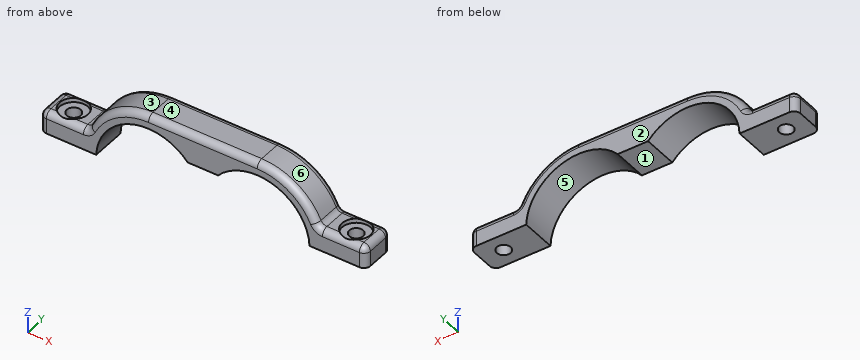
from build123d import *

# Parameters (mm, degrees)
BOSS_EXTRU_1_DEPTH      = 8
ESQUISSE2_R             = 1.6
ENL_V_MAT_EXTRU_1_DEPTH = 42.011614209
ENL_V_START             = -4
ESQUISSE3_R             = 3.25
ENL_V_MAT_EXTRU_2_DEPTH = 38.011614209
CONG_1_R                = 1.5


with BuildPart() as part:
    # Esquisse1 → Boss.-Extru.1 (new body)
    with BuildSketch(Plane(origin=(0, 0, 0), x_dir=(1, 0, 0), z_dir=(0, 1, 0))):
        with BuildLine():
            Line((-37.5, -0.5), (-24.539622087, -0.5))
            ThreePointArc((-24.539622087, -0.5), (-16.544164933, -11.351089375), (-3.488757022, -8))
            Line((-3.488757022, -8), (3.488757022, -8))
            ThreePointArc((3.488757022, -8), (16.544164933, -11.351089375), (24.539622087, -0.5))
            Line((24.539622087, -0.5), (37.5, -0.5))
            Line((37.5, -0.5), (37.5, -5.5))
            Line((37.5, -5.5), (26.509014955, -5.5))
            ThreePointArc((26.509014955, -5.5), (20.977248964, -12.435382986), (12.5, -15.05))
            Line((12.5, -15.05), (-12.5, -15.05))
            ThreePointArc((-12.5, -15.05), (-20.977248964, -12.435382986), (-26.509014955, -5.5))
            Line((-26.509014955, -5.5), (-37.5, -5.5))
            Line((-37.5, -5.5), (-37.5, -0.5))
        make_face()
    extrude(amount=BOSS_EXTRU_1_DEPTH)

    # Esquisse2 → Enlèv. mat.-Extru.1 (cut, through all)
    with BuildSketch(Plane(origin=(0, 0, 0.5), x_dir=(-1, 0, 0), z_dir=(0, 0, -1))):
        with Locations((32.5, 4)):
            Circle(ESQUISSE2_R)
        with Locations((-32.5, 4)):
            Circle(ESQUISSE2_R)
    extrude(amount=-ENL_V_MAT_EXTRU_1_DEPTH, mode=Mode.SUBTRACT)

    # Esquisse3 → Enlèv. mat.-Extru.2 (cut, through all)
    with BuildSketch(Plane(origin=(0, 0, 0.5), x_dir=(-1, 0, 0), z_dir=(0, 0, -1)).offset(ENL_V_START)):
        with Locations((32.5, 4)):
            Circle(ESQUISSE3_R)
        with Locations((-32.5, 4)):
            Circle(ESQUISSE3_R)
    extrude(amount=-ENL_V_MAT_EXTRU_2_DEPTH, mode=Mode.SUBTRACT)

    # Congé1
    # the kernel refuses this fillet: 1.5 mm, written as the material it adds along each edge
    with BuildSketch(Plane(origin=(26.509014955, 0, 5.5), x_dir=(-0.3943977660181821, 0, 0.9189398251027471), z_dir=(0, 1, 0))) as cong_1_piece_1:
        with BuildLine():
            CenterArc((0.988849381, 1.499265395), CONG_1_R, 203.228419566, 64.978347937)
            Line((-0.389560356, 0.907668746), (0, 0))
            ThreePointArc((0, 0), (0.470955164, 0.007370535), (0.941910328, 0))
        make_face()
    extrude(amount=8)
    with BuildSketch(Plane(origin=(-26.509014955, 0, 5.5), x_dir=(0.3943977660181821, 0, 0.9189398251027471), z_dir=(0, 1, 0))) as cong_1_piece_2:
        with BuildLine():
            CenterArc((0.988849381, -1.499265395), CONG_1_R, 91.793232497, 64.978347937)
            Line((-0.389560356, -0.907668746), (0, 0))
            ThreePointArc((0, 0), (0.470955164, -0.007370535), (0.941910328, 0))
        make_face()
    extrude(amount=8)
    # the kernel refuses this fillet: 1.5 mm, written as the material it takes off along each edge
    with BuildSketch(Plane(origin=(37.5, 0, -3.25), x_dir=(-1, 0, 0), z_dir=(0, 0, 1)), Plane(origin=(-37.5, 0, 9.25), x_dir=(1, 0, 0), z_dir=(0, 0, -1))) as cong_1_2_piece_1:
        with BuildLine():
            CenterArc((CONG_1_R, -CONG_1_R), CONG_1_R, 90, 90)
            Line((0, -CONG_1_R), (0, 0))
            Line((0, 0), (CONG_1_R, 0))
        make_face()
    extrude(amount=12.5, mode=Mode.SUBTRACT)
    with BuildSketch(Plane(origin=(-37.5, 8, 9.25), x_dir=(1, 0, 0), z_dir=(0, 0, -1)), Plane(origin=(37.5, 8, -3.25), x_dir=(-1, 0, 0), z_dir=(0, 0, 1))) as cong_1_2_piece_2:
        with BuildLine():
            CenterArc((CONG_1_R, CONG_1_R), CONG_1_R, 180, 90)
            Line((0, CONG_1_R), (0, 0))
            Line((0, 0), (CONG_1_R, 0))
        make_face()
    extrude(amount=12.5, mode=Mode.SUBTRACT)
    with BuildSketch(Plane(origin=(37.5, -3.75, 5.5), x_dir=(0, 0, -1), z_dir=(0, 1, 0)), Plane(origin=(-37.5, -3.75, 5.5), x_dir=(1, 0, 0), z_dir=(0, 1, 0))) as cong_1_2_piece_3:
        with BuildLine():
            CenterArc((CONG_1_R, CONG_1_R), CONG_1_R, 180, 90)
            Line((0, CONG_1_R), (0, 0))
            Line((0, 0), (CONG_1_R, 0))
        make_face()
    extrude(amount=15.5, mode=Mode.SUBTRACT)
    # the kernel refuses this fillet: 1.5 mm, written as the material it takes off along each edge
    with BuildSketch(Plane(origin=(36, 6.5, 4), x_dir=(0, 0, 1), z_dir=(0, 1, 0))) as cong_1_3_piece_1_section:
        Polygon((0, 0), (CONG_1_R, 0), (CONG_1_R, CONG_1_R), (0, CONG_1_R), align=None)
    cong_1_3_piece_1 = extrude(amount=CONG_1_R, mode=Mode.PRIVATE)
    cong_1_3_piece_1 = cong_1_3_piece_1 - Plane(origin=(36, 6.5, 4), x_dir=(-0.7071067811865475, 0, -0.7071067811865475), z_dir=(0, 1, 0)) * Sphere(CONG_1_R, mode=Mode.PRIVATE)
    add(cong_1_3_piece_1, mode=Mode.SUBTRACT)
    with BuildSketch(Plane(origin=(-36, 6.5, 4), x_dir=(0, 0, 1), z_dir=(0, 1, 0))) as cong_1_3_piece_2_section:
        Polygon((0, 0), (CONG_1_R, 0), (CONG_1_R, -CONG_1_R), (0, -CONG_1_R), align=None)
    cong_1_3_piece_2 = extrude(amount=CONG_1_R, mode=Mode.PRIVATE)
    cong_1_3_piece_2 = cong_1_3_piece_2 - Plane(origin=(-36, 6.5, 4), x_dir=(0.7071067811865475, 0, -0.7071067811865475), z_dir=(0, 1, 0)) * Sphere(CONG_1_R, mode=Mode.PRIVATE)
    add(cong_1_3_piece_2, mode=Mode.SUBTRACT)
    with BuildSketch(Plane(origin=(-36, 1.5, 4), x_dir=(0, 0, 1), z_dir=(0, -1, 0))) as cong_1_3_piece_3_section:
        Polygon((0, 0), (CONG_1_R, 0), (CONG_1_R, CONG_1_R), (0, CONG_1_R), align=None)
    cong_1_3_piece_3 = extrude(amount=CONG_1_R, mode=Mode.PRIVATE)
    cong_1_3_piece_3 = cong_1_3_piece_3 - Plane(origin=(-36, 1.5, 4), x_dir=(0.7071067811865475, 0, -0.7071067811865475), z_dir=(0, -1, 0)) * Sphere(CONG_1_R, mode=Mode.PRIVATE)
    add(cong_1_3_piece_3, mode=Mode.SUBTRACT)
    with BuildSketch(Plane(origin=(36, 1.5, 4), x_dir=(0, 0, 1), z_dir=(0, -1, 0))) as cong_1_3_piece_4_section:
        Polygon((0, 0), (CONG_1_R, 0), (CONG_1_R, -CONG_1_R), (0, -CONG_1_R), align=None)
    cong_1_3_piece_4 = extrude(amount=CONG_1_R, mode=Mode.PRIVATE)
    cong_1_3_piece_4 = cong_1_3_piece_4 - Plane(origin=(36, 1.5, 4), x_dir=(-0.7071067811865475, 0, -0.7071067811865475), z_dir=(0, -1, 0)) * Sphere(CONG_1_R, mode=Mode.PRIVATE)
    add(cong_1_3_piece_4, mode=Mode.SUBTRACT)
    with BuildSketch(Plane(origin=(36, 0, 5.5), x_dir=(0, 0, -1), z_dir=(-1, 0, 0)), Plane(origin=(-27.496749648, 0, 5.5), x_dir=(0, 0, -1), z_dir=(-1, 0, 0))) as cong_1_3_piece_5:
        with BuildLine():
            CenterArc((CONG_1_R, -CONG_1_R), CONG_1_R, 90, 90)
            Line((0, -CONG_1_R), (0, 0))
            Line((0, 0), (CONG_1_R, 0))
        make_face()
    extrude(amount=8.503250352, mode=Mode.SUBTRACT)
    with BuildSketch(Plane(origin=(12.5, 0, 0), x_dir=(0.9061480149752484, 0, 0.4229607250755286), z_dir=(0.4229607250755286, 0, -0.9061480149752484))) as cong_1_3_piece_6:
        with BuildLine():
            CenterArc((15.05 - CONG_1_R, -CONG_1_R), CONG_1_R, 0, 90)
            Line((15.05 - CONG_1_R, 0), (15.05, 0))
            Line((15.05, 0), (15.05, -CONG_1_R))
        make_face()
    revolve(axis=Axis((12.5, 0, 0), (0, -1, 0)), revolution_arc=64.978347937, mode=Mode.SUBTRACT)
    with BuildSketch(Plane(origin=(12.5, 0, 15.05), x_dir=(0, 0, -1), z_dir=(-1, 0, 0)), Plane(origin=(12.5, 8, 15.05), x_dir=(0, -1, 0), z_dir=(-1, 0, 0))) as cong_1_3_piece_7:
        with BuildLine():
            CenterArc((CONG_1_R, -CONG_1_R), CONG_1_R, 90, 90)
            Line((0, -CONG_1_R), (0, 0))
            Line((0, 0), (CONG_1_R, 0))
        make_face()
    extrude(amount=25, mode=Mode.SUBTRACT)
    with BuildSketch(Plane(origin=(-12.5, 0, 0), x_dir=(0, 0, 1), z_dir=(1, 0, 0))) as cong_1_3_piece_8:
        with BuildLine():
            CenterArc((15.05 - CONG_1_R, -CONG_1_R), CONG_1_R, 0, 90)
            Line((15.05, -CONG_1_R), (15.05, 0))
            Line((15.05, 0), (15.05 - CONG_1_R, 0))
        make_face()
    revolve(axis=Axis((-12.5, 0, 0), (0, -1, 0)), revolution_arc=64.978347937, mode=Mode.SUBTRACT)
    with BuildSketch(Plane(origin=(-27.496749648, 8, 5.5), x_dir=(0, 0, -1), z_dir=(-1, 0, 0)), Plane(origin=(36, 8, 5.5), x_dir=(0, 0, -1), z_dir=(-1, 0, 0))) as cong_1_3_piece_9:
        with BuildLine():
            CenterArc((CONG_1_R, CONG_1_R), CONG_1_R, 180, 90)
            Line((0, CONG_1_R), (0, 0))
            Line((0, 0), (CONG_1_R, 0))
        make_face()
    extrude(amount=8.503250352, mode=Mode.SUBTRACT)
    with BuildSketch(Plane(origin=(-12.5, 8, 0), x_dir=(0, 0, 1), z_dir=(1, 0, 0))) as cong_1_3_piece_10:
        with BuildLine():
            CenterArc((15.05 - CONG_1_R, CONG_1_R), CONG_1_R, 270, 90)
            Line((15.05, CONG_1_R), (15.05, 0))
            Line((15.05, 0), (15.05 - CONG_1_R, 0))
        make_face()
    revolve(axis=Axis((-12.5, 8, 0), (0, -1, 0)), revolution_arc=64.978347937, mode=Mode.SUBTRACT)
    with BuildSketch(Plane(origin=(12.5, 8, 0), x_dir=(0.9061480149752484, 0, 0.4229607250755286), z_dir=(0.4229607250755286, 0, -0.9061480149752484))) as cong_1_3_piece_11:
        with BuildLine():
            CenterArc((15.05 - CONG_1_R, CONG_1_R), CONG_1_R, 270, 90)
            Line((15.05 - CONG_1_R, 0), (15.05, 0))
            Line((15.05, 0), (15.05, CONG_1_R))
        make_face()
    revolve(axis=Axis((12.5, 8, 0), (0, -1, 0)), revolution_arc=64.978347937, mode=Mode.SUBTRACT)
    with BuildSketch(Plane(origin=(27.496749648, 8, 7), x_dir=(-0.9061480149752484, 0, -0.4229607250755287), z_dir=(-0.4229607250755287, 0, 0.9061480149752484))) as cong_1_3_piece_12:
        with BuildLine():
            CenterArc((1.5 + CONG_1_R, CONG_1_R), CONG_1_R, 180, 90)
            Line((1.5, CONG_1_R), (1.5, 0))
            Line((1.5, 0), (1.5 + CONG_1_R, 0))
        make_face()
    revolve(axis=Axis((27.496749648, 8, 7), (0, -1, 0)), revolution_arc=64.978347937, mode=Mode.SUBTRACT)
    with BuildSketch(Plane(origin=(-27.496749648, 8, 7), x_dir=(0.9061480149752487, 0, -0.42296072507552823), z_dir=(0.42296072507552823, 0, 0.9061480149752487))) as cong_1_3_piece_13:
        with BuildLine():
            CenterArc((1.5 + CONG_1_R, -CONG_1_R), CONG_1_R, 90, 90)
            Line((1.5, -CONG_1_R), (1.5, 0))
            Line((1.5, 0), (1.5 + CONG_1_R, 0))
        make_face()
    revolve(axis=Axis((-27.496749648, 8, 7), (0, 1, 0)), revolution_arc=64.978347937, mode=Mode.SUBTRACT)
    with BuildSketch(Plane(origin=(-27.496749648, 0, 7), x_dir=(0.9061480149752487, 0, -0.42296072507552823), z_dir=(0.42296072507552823, 0, 0.9061480149752487))) as cong_1_3_piece_14:
        with BuildLine():
            CenterArc((1.5 + CONG_1_R, CONG_1_R), CONG_1_R, 180, 90)
            Line((1.5, CONG_1_R), (1.5, 0))
            Line((1.5, 0), (1.5 + CONG_1_R, 0))
        make_face()
    revolve(axis=Axis((-27.496749648, 0, 7), (0, 1, 0)), revolution_arc=64.978347937, mode=Mode.SUBTRACT)
    with BuildSketch(Plane(origin=(27.496749648, 0, 7), x_dir=(-0.9061480149752484, 0, -0.4229607250755287), z_dir=(-0.4229607250755287, 0, 0.9061480149752484))) as cong_1_3_piece_15:
        with BuildLine():
            CenterArc((1.5 + CONG_1_R, -CONG_1_R), CONG_1_R, 90, 90)
            Line((1.5, -CONG_1_R), (1.5, 0))
            Line((1.5, 0), (1.5 + CONG_1_R, 0))
        make_face()
    revolve(axis=Axis((27.496749648, 0, 7), (0, -1, 0)), revolution_arc=64.978347937, mode=Mode.SUBTRACT)


solid = part.part
Design review of the part built by this model. Coordinates are the model's own, in mm. Face numbers are marked on the shaded views. A direction names the side the tool comes from. Round coordinates to 2 decimals unless told otherwise and drop trailing zeros. Loops run counter-clockwise (first coordinate to the right, second up) from the corner with the lowest first, then second, coordinate; pieces in that order, holes last. Notation, with made-up numbers: (64.5, 16.25) -> (82.5, 16.25) arc R7 cw to (82.5, 24.25) -> close; hole circle Ø8 at (-35, 51.25). An arc over 180 degrees is marked (long way). Use one line per item in the form item = value. Start each with the question number.
Q1. Machinability: for the marked faces 1 and 2, which of the approach directions +Z, -Z, +X, -X, +Y, -Y give a long, thin tool a straight path to every point of the face, cutting with its end or side? Answer none if there is none.
Q2. Wall thickness on line 1 along X through (y, z) = (1.5, 9.25); line 2 along X through (y, z) = (4, 5.1); line 3 along X through (y, z) = (4, 10.5): over which ranges is each line inside the solid? List them lowest first. Write a range as [from, to].
Q3. For pin 1 Ø1.5 at (x, y) = (-29, 3) entering from +Z; pin 2 Ø3.5 at (x, y) = (0.5, 6) entering from -Z; pin 3 Ø3 at (y, z) = (2, 12.5) entering from -X, all flat-tipped, find the tip position at first contact; note any pin that passes through.
Q4. We need section A-A on y = 4. State how many separate pieces and enclosed holes the cut face has, then the cut area to 3 significant figures.
Q5. We need section B-B on x = -32.5. Give the boundary of the cut face in (y, z), then the cut area to 3 significant figures.
Q6. We need section C-C on x = 1.5. Give the boundary of the cut face in (y, z).
Q7. Draft analysis for pull direction X (two halves, no side actions). For the marked faces 3, 4, 5 and 6, state which applies: +X half, -X half, draft (parallel to the pull), parting line (faces both ways), or undercut.
Calculated:
q1.face_1 = -Z, +Y, -Y
q1.face_2 = +Z, -Z, +X, -X, +Y
q2.line_1 = [-24.37, -20.22], [-4.78, 4.78], [20.22, 24.37]
q2.line_2 = [-37.02, -35.75], [-29.25, -23.42], [23.42, 29.25], [35.75, 37.02]
q2.line_3 = [-23.28, -18.41], [-6.59, 6.59], [18.41, 23.28]
q3.pin_1 = 5.5
q3.pin_2 = 8
q3.pin_3 = -22.77
q4.separate_pieces = 3
q4.enclosed_holes = 0
q4.area = 314 mm²
q5.outline = (0, 0.5) -> (2.4, 0.5) -> (2.4, 4.5) -> (0.75, 4.5) -> (0.75, 5.3) arc R1.5 ccw to (0, 4) -> close; (5.6, 0.5) -> (8, 0.5) -> (8, 4) arc R1.5 ccw to (7.25, 5.3) -> (7.25, 4.5) -> (5.6, 4.5) -> close
q5.area = 19.8 mm²
q6.outline = (0, 8) -> (8, 8) -> (8, 13.55) arc R1.5 ccw to (6.5, 15.05) -> (1.5, 15.05) arc R1.5 ccw to (0, 13.55) -> close
q7.face_3 = -X half
q7.face_4 = draft
q7.face_5 = undercut
q7.face_6 = +X half
